Verification items for the finished model (mm, model axes). A direction names the side the tool comes from. Coordinates: 2 decimals unless noted, no trailing zeros. Write each loop counter-clockwise with the first axis right and the second up, starting at its lowest first coordinate (ties: lowest second). Pieces come first, ordered by that corner, then holes. Notation, with made-up numbers: (19.25, 71) -> (65.25, 71) arc R18 cw to (65.25, 89) -> close; hole circle Ø7 at (36.25, 45). An arc over 180 degrees is marked (long way). Answer in a Markdown table with one row per item.
```python
from build123d import *

# Parameters (mm, degrees)
BOSS_EXTRUDE1_DEPTH = 5
BOSS_EXTRUDE2_DEPTH = 13
CUT_EXTRUDE1_DEPTH  = 5
CUT_EXTRUDE2_START  = -5
CUT_EXTRUDE2_DEPTH  = 5
SKETCH5_R           = 2.4
CUT_EXTRUDE3_DEPTH  = 64.984373092
CUT_EXTRUDE4_DEPTH  = 3
SKETCH7_R           = 14
CUT_EXTRUDE5_DEPTH  = 1
CUT_EXTRUDE6_START  = -1
SKETCH8_R           = 14
CUT_EXTRUDE6_DEPTH  = 1
SKETCH9_R           = 4
CUT_EXTRUDE7_DEPTH  = 64.788713735
SKETCH10_R          = 12.55
SKETCH10_R_2        = 12.5
CUT_EXTRUDE8_DEPTH  = 0.5
SKETCH11_R          = 11
SKETCH11_R_2        = 10.95
CUT_EXTRUDE9_DEPTH  = 0.5
SKETCH12_R          = 5.5
SKETCH12_R_2        = 5.45
CUT_EXTRUDE10_DEPTH = 0.5
CUT_EXTRUDE11_START = -0.5
SKETCH13_R          = 5.5
SKETCH13_R_2        = 5.45
CUT_EXTRUDE11_DEPTH = 0.5
CUT_EXTRUDE12_START = -0.5
SKETCH14_R          = 12.55
SKETCH14_R_2        = 12.5
CUT_EXTRUDE12_DEPTH = 0.5
CUT_EXTRUDE13_START = -0.5
SKETCH15_R          = 11
SKETCH15_R_2        = 10.95
CUT_EXTRUDE13_DEPTH = 0.5


with BuildPart() as part:
    # Sketch1 → Boss-Extrude1 (new body)
    with BuildSketch(Plane(origin=(0, 0, 0), x_dir=(1, 0, 0), z_dir=(0, 1, 0))):
        Polygon((0, -3), (0, -10), (3, -13), (52, -13), (55, -10), (55, -3), (52, 0), (3, 0), align=None)
    extrude(amount=BOSS_EXTRUDE1_DEPTH)

    # Sketch2 → Boss-Extrude2 (add)
    with BuildSketch(Plane.XY.offset(13)):
        with BuildLine():
            Line((12.5, 15), (12.5, 0))
            Line((12.5, 0), (42.5, 0))
            Line((42.5, 0), (42.5, 15))
            ThreePointArc((42.5, 15), (27.5, 30), (12.5, 15))
        make_face()
    extrude(amount=-BOSS_EXTRUDE2_DEPTH)

    # Sketch3 → Cut-Extrude1 (cut)
    with BuildSketch(Plane.XY.offset(13)):
        with BuildLine():
            Line((14.5, 7.516685226), (14.5, 0))
            Line((14.5, 0), (14.5, -1))
            Line((14.5, -1), (40.5, -1))
            Line((40.5, -1), (40.5, 0))
            Line((40.5, 0), (40.5, 7.516685226))
            ThreePointArc((40.5, 7.516685226), (27.5, 0), (14.5, 7.516685226))
        make_face()
    extrude(amount=-CUT_EXTRUDE1_DEPTH, mode=Mode.SUBTRACT)

    # Sketch4 → Cut-Extrude2 (cut)
    with BuildSketch(Plane(origin=(0, 0, 0), x_dir=(-1, 0, 0), z_dir=(0, 0, -1)).offset(CUT_EXTRUDE2_START)):
        with BuildLine():
            Line((-40.5, 7.516685226), (-40.5, -2.151111231))
            Line((-40.5, -2.151111231), (-14.5, -2.151111231))
            Line((-14.5, -2.151111231), (-14.5, 7.516685226))
            ThreePointArc((-14.5, 7.516685226), (-27.5, 0), (-40.5, 7.516685226))
        make_face()
    extrude(amount=CUT_EXTRUDE2_DEPTH, mode=Mode.SUBTRACT)

    # Sketch5 → Cut-Extrude3 (cut, through all)
    with BuildSketch(Plane.XZ):
        with Locations(Location((6.5, 6.5, 0), (0, 0, 270))):
            Circle(SKETCH5_R)
        with Locations(Location((48.5, 6.5, 0), (0, 0, 90))):
            Circle(SKETCH5_R)
    extrude(amount=-CUT_EXTRUDE3_DEPTH, mode=Mode.SUBTRACT)

    # Sketch6 → Cut-Extrude4 (cut)
    with BuildSketch(Plane.XZ):
        Polygon((12.5, 2), (12.5, 11), (3.828427125, 11), (2, 9.171572875), (2, 3.828427125), (3.828427125, 2), align=None)
        Polygon((51.171572875, 2), (42.5, 2), (42.5, 11), (51.171572875, 11), (53, 9.171572875), (53, 3.828427125), align=None)
    extrude(amount=-CUT_EXTRUDE4_DEPTH, mode=Mode.SUBTRACT)

    # Sketch7 → Cut-Extrude5 (cut)
    with BuildSketch(Plane.XY.offset(13)):
        with Locations((27.5, 15)):
            Circle(SKETCH7_R)
    extrude(amount=-CUT_EXTRUDE5_DEPTH, mode=Mode.SUBTRACT)

    # Sketch8 → Cut-Extrude6 (cut)
    with BuildSketch(Plane(origin=(0, 0, 0), x_dir=(-1, 0, 0), z_dir=(0, 0, -1)).offset(CUT_EXTRUDE6_START)):
        with Locations(Location((-27.5, 15, 0), (0, 0, 180))):
            Circle(SKETCH8_R)
    extrude(amount=CUT_EXTRUDE6_DEPTH, mode=Mode.SUBTRACT)

    # Sketch9 → Cut-Extrude7 (cut, through all)
    with BuildSketch(Plane.XY.offset(12)):
        with Locations((27.5, 15)):
            Circle(SKETCH9_R)
    extrude(amount=-CUT_EXTRUDE7_DEPTH, mode=Mode.SUBTRACT)

    # Sketch10 → Cut-Extrude8 (cut)
    with BuildSketch(Plane.XY.offset(12)):
        with Locations((27.5, 15)):
            Circle(SKETCH10_R)
        with Locations((27.5, 15)):
            Circle(SKETCH10_R_2, mode=Mode.SUBTRACT)
    extrude(amount=-CUT_EXTRUDE8_DEPTH, mode=Mode.SUBTRACT)

    # Sketch11 → Cut-Extrude9 (cut)
    with BuildSketch(Plane.XY.offset(12)):
        with Locations((27.5, 15)):
            Circle(SKETCH11_R)
        with Locations((27.5, 15)):
            Circle(SKETCH11_R_2, mode=Mode.SUBTRACT)
    extrude(amount=-CUT_EXTRUDE9_DEPTH, mode=Mode.SUBTRACT)

    # Sketch12 → Cut-Extrude10 (cut)
    with BuildSketch(Plane.XY.offset(12)):
        with Locations((27.5, 15)):
            Circle(SKETCH12_R)
        with Locations((27.5, 15)):
            Circle(SKETCH12_R_2, mode=Mode.SUBTRACT)
    extrude(amount=-CUT_EXTRUDE10_DEPTH, mode=Mode.SUBTRACT)

    # Sketch13 → Cut-Extrude11 (cut)
    with BuildSketch(Plane(origin=(0, 0, 1), x_dir=(-1, 0, 0), z_dir=(0, 0, -1)).offset(CUT_EXTRUDE11_START)):
        with Locations(Location((-27.5, 15, 0), (0, 0, 180))):
            Circle(SKETCH13_R)
        with Locations(Location((-27.5, 15, 0), (0, 0, 180))):
            Circle(SKETCH13_R_2, mode=Mode.SUBTRACT)
    extrude(amount=CUT_EXTRUDE11_DEPTH, mode=Mode.SUBTRACT)

    # Sketch14 → Cut-Extrude12 (cut)
    with BuildSketch(Plane(origin=(0, 0, 1), x_dir=(-1, 0, 0), z_dir=(0, 0, -1)).offset(CUT_EXTRUDE12_START)):
        with Locations(Location((-27.5, 15, 0), (0, 0, 180))):
            Circle(SKETCH14_R)
        with Locations(Location((-27.5, 15, 0), (0, 0, 180))):
            Circle(SKETCH14_R_2, mode=Mode.SUBTRACT)
    extrude(amount=CUT_EXTRUDE12_DEPTH, mode=Mode.SUBTRACT)

    # Sketch15 → Cut-Extrude13 (cut)
    with BuildSketch(Plane(origin=(0, 0, 1), x_dir=(-1, 0, 0), z_dir=(0, 0, -1)).offset(CUT_EXTRUDE13_START)):
        with Locations(Location((-27.5, 15, 0), (0, 0, 180))):
            Circle(SKETCH15_R)
        with Locations(Location((-27.5, 15, 0), (0, 0, 180))):
            Circle(SKETCH15_R_2, mode=Mode.SUBTRACT)
    extrude(amount=CUT_EXTRUDE13_DEPTH, mode=Mode.SUBTRACT)


solid = part.part
```
1. Release check for a two-part mould opening along X. For faces 1 (the face through (27.83, 29.996, 6.591)), 2 (the face through (22, 13, 12)), 3 (the face through (2, 1, 7)), 4 (the face through (1, 2, 11)) record: released by +X, released by -X, zero draft, split by the parting line, or undercut.
Findings below:
| item | result |
|---|---|
| face 1 | split by the parting line |
| face 2 | undercut |
| face 3 | undercut |
| face 4 | released by -X |
2. Sectioned sample at B-B, the plane z = 6.5. Record the cut outline in (x, y).
Findings below:
| item | result |
|---|---|
| outline | (0, 0) -> (2, 0) -> (2, 3) -> (4.1, 3) -> (4.1, 5) -> (0, 5) -> close; (8.9, 3) -> (12.5, 3) -> (12.5, 0) -> (42.5, 0) -> (42.5, 3) -> (46.1, 3) -> (46.1, 5) -> (42.5, 5) -> (42.5, 15) arc R15 ccw to (12.5, 15) -> (12.5, 5) -> (8.9, 5) -> close; (50.9, 3) -> (53, 3) -> (53, 0) -> (55, 0) -> (55, 5) -> (50.9, 5) -> close; hole circle Ø8 at (27.5, 15) |
3. Access from +Z, -Z, +X, -X, +Y, -Y to the whole of each face (thin tool, end or side, straight path). Record for faces 5 (the face through (52.1, 1.48, 2.93)), 6 (the face through (12.5, 10, 7)), 7 (the face through (26, 19, 12)), 8 (the face through (2, 2, 1)).
Findings below:
| item | result |
|---|---|
| face 5 | -Y |
| face 6 | +Z, -Z, -X, +Y |
| face 7 | +Z |
| face 8 | -Z, -X, +Y, -Y |
4. Sectioned sample at A-A, the plane x = 48.5. Record the cut outline in (y, z).
Findings below:
| item | result |
|---|---|
| outline | (0, 0) -> (5, 0) -> (5, 4.1) -> (3, 4.1) -> (3, 2) -> (0, 2) -> close; (0, 11) -> (3, 11) -> (3, 8.9) -> (5, 8.9) -> (5, 13) -> (0, 13) -> close |
5. Go/stop test with flat-tipped pins: pin 1 (5.5 mm diameter, centred on x = 48.5, z = 6.5, fed in from +Y); pin 2 (1.5 mm diameter, centred on x = 11.5, z = 5.5, fed in from -Y); pin 3 (3 mm diameter, centred on y = 19, z = 11.5, fed in from -X); pin 4 (1 mm diameter, centred on x = 40.5, y = 24, fed in from +Z). Record where each tip stops, or that it passes through.
Findings below:
| item | result |
|---|---|
| pin 1 | stops at y = 5 |
| pin 2 | stops at y = 3 |
| pin 3 | stops at x = 12.71 |
| pin 4 | passes through |
6. Material ranges on probe 1 along X at (y, z) = (4.45, 6.5); probe 2 along Z at (x, y) = (48.5, 4.45); probe 3 along Y at (x, z) = (10, 7), recorded low to high. Write a range as from..to.
Findings below:
| item | result |
|---|---|
| probe 1 | x = 0..4.1, 8.9..46.1, 50.9..55 |
| probe 2 | z = 0..4.1, 8.9..13 |
| probe 3 | y = 3..5 |
